Could you check a few things on this model? Use its own coordinates, in mm. A direction names the side the tool comes from. Coordinates: 2 decimals unless noted, no trailing zeros. Write each loop counter-clockwise with the first axis right and the second up, starting at its lowest first coordinate (ties: lowest second). Pieces come first, ordered by that corner, then holes.
```python
from build123d import *

# Parameters (mm, degrees)
F0_W     = 16
F0_H     = 16
F0_W_2   = 10
F0_H_2   = 10
F1_DEPTH = 24
F2_W     = 16
F2_H     = 16
F2_W_2   = 10
F2_H_2   = 10
F3_DEPTH = 16
F4_W     = 3
F4_H     = 5
F5_DEPTH = 25
F6_W     = 3
F6_H     = 16
F7_DEPTH = 16
F8_R     = 1.5
F9_DEPTH = 13.501


with BuildPart() as f1:
    # F0 (on Right) → F1 (new body)
    with BuildSketch(Plane.YZ):
        Rectangle(F0_W, F0_H)
        Rectangle(F0_W_2, F0_H_2, mode=Mode.SUBTRACT)
    extrude(amount=F1_DEPTH)

    # F2 (on face) → F3 (join)
    with BuildSketch(Plane.XY.offset(8)):
        with Locations((-8, 0)):
            Rectangle(F2_W, F2_H)
        with Locations((-8, 0)):
            Rectangle(F2_W_2, F2_H_2, mode=Mode.SUBTRACT)
    extrude(amount=-F3_DEPTH)

    # F4 (on face) → F5 (cut)
    with BuildSketch(Plane.XY.offset(8)):
        with Locations((-14.5, 0)):
            Rectangle(F4_W, F4_H)
    extrude(amount=-F5_DEPTH, mode=Mode.SUBTRACT)

    # F6 (on face) → F7 (join)
    with BuildSketch(Plane(origin=(-16, 0, 0), x_dir=(0, -1, 0), z_dir=(-1, 0, 0))):
        with Locations((-4, 0)):
            Rectangle(F6_W, F6_H)
        with Locations((4, 0)):
            Rectangle(F6_W, F6_H)
    extrude(amount=F7_DEPTH)

    # F8 (on face) → F9 (cut, through all)
    with BuildSketch(Plane.XZ.offset(5.5)):
        with Locations((-24, 0)):
            Circle(F8_R)
    extrude(amount=-F9_DEPTH, mode=Mode.SUBTRACT)


solid = f1.part
```
Item 1: I want a section at D-D, the plane z = 2. List the corners of the cut face in (x, y) for me, then the cut area to 3 significant figures.
Item 2: Will these pins go through, and if not, where does the flat tip stop? pin 1 Ø1.5 at (y, z) = (-4, -2.5) entering from +X; pin 2 Ø5 at (x, z) = (-24, 0) entering from +Y; pin 3 Ø1.8 at (x, z) = (-24, 0) entering from +Y.
Item 3: If I drill on line 1 along Y through (x, z) = (-8.5, 6.75); line 2 along Z through (x, y) = (-24, -3.25); line 3 along X through (y, z) = (-3.5, 6.25), over which ranges is the centre line in solid material (lowest first)?
Item 4: If we mould it in two halves opening along Z, with no side actions, what happens to faces 1 (the flat face through (12, 0, -5)), 2 (the flat face through (12, 5, 0)), 3 (the flat face through (24, -0.1, 5.4))? For each: released by +Z, released by -Z, zero draft, split by the parting line, or undercut.
Item 5: Which directions (+Z, -Z, +X, -X, +Y, -Y) give clear straight access to the entire face, cutting with the end or side of a thin tool? Please do faces 4 (the flat face through (-16, -7, 0)), 5 (the flat face through (-13, 4, 0)), 6 (the flat face through (-22, 5.5, 0)), 7 (the flat face through (-22, 2.5, 0)), 8 (the flat face through (12, 0, 5)).
Item 6: I want a section at C-C, the plane x = 10.5. List the corners of the cut face in (y, z) for me, then the cut area to 3 significant figures.
Item 7: I want a section at A-A, the plane y = 3.25. List the corners of the cut face in (x, z) for me.
Item 8: I want a section at B-B, the plane x = -24. List the corners of the cut face in (y, z) for me.
Taken from the geometry:
1. outline: (-32, -5.5) - (-16, -5.5) - (-16, -8) - (24, -8) - (24, -5) - (0, -5) - (0, 5) - (24, 5) - (24, 8) - (-16, 8) - (-16, 5.5) - (-32, 5.5) - (-32, 2.5) - (-13, 2.5) - (-13, 5) - (-3, 5) - (-3, -5) - (-13, -5) - (-13, -2.5) - (-32, -2.5) - close
1. area: 381 mm2
2. pin 1: stops at x = 0
2. pin 2: stops at y = 5.5
2. pin 3: passes through
3. line 1: y = -8 to -5, 5 to 8
3. line 2: z = -8 to -1.5, 1.5 to 8
3. line 3: x = -32 to -13, -3 to 24
4. face 1: undercut
4. face 2: undercut
4. face 3: zero draft
5. face 4: +Z, -Z, -X, -Y
5. face 5: +Z, -Z
5. face 6: +Z, -Z, -X, +Y
5. face 7: +Z, -Z, -X
5. face 8: +X
6. outline: (-8, -8) - (8, -8) - (8, 8) - (-8, 8) - close; hole (-5, -5) - (5, -5) - (5, 5) - (-5, 5) - close
6. area: 156 mm2
7. outline: (-32, -8) - (-13, -8) - (-13, 8) - (-32, 8) - close; (-3, -8) - (24, -8) - (24, -5) - (0, -5) - (0, 5) - (24, 5) - (24, 8) - (-3, 8) - close; hole circle Ø3 at (-24, 0)
8. outline: (-5.5, -8) - (-2.5, -8) - (-2.5, -1.5) - (-5.5, -1.5) - close; (-5.5, 1.5) - (-2.5, 1.5) - (-2.5, 8) - (-5.5, 8) - close; (2.5, -8) - (5.5, -8) - (5.5, -1.5) - (2.5, -1.5) - close; (2.5, 1.5) - (5.5, 1.5) - (5.5, 8) - (2.5, 8) - close
